Work out the finished part from the listing and answer in its coordinate system (mm). Round coordinates to 2 decimals unless told otherwise and drop trailing zeros. Order: outer loops, then holes, each group sorted by start corner. A loop starts at its lowest first (then second) coordinate and runs counter-clockwise, first axis right, second up. Notation, with made-up numbers: (89.25, -21.5) - (128.25, -21.5) arc R19 cw to (128.25, 8.5) - close; hole circle Ø3 at (61, 45.25). An arc over 180 degrees is marked (long way). Answer in a Markdown table with one row per item.
from build123d import *

# Parameters (mm, degrees)
SKETCH1_R               = 12.5
BOSS_EXTRUDE1_DEPTH     = 900
CHAMFER1_SIZE           = 1
SKETCH2_R               = 3.3
CUT_EXTRUDE1_DEPTH      = 40.5
CUT_EXTRUDE1_DEPTH_BACK = 7


with BuildPart() as part:
    # Sketch1 → Boss-Extrude1 (new body)
    with BuildSketch(Plane.XY):
        with Locations((0, 33)):
            Circle(SKETCH1_R)
        Polygon((-27.5, 0), (-4.75, 0), (-4.75, 6.5), (4.75, 6.5), (4.75, 0), (27.5, 0), (27.5, 6), (10.75, 6), (2.089745962, 21), (-2.089745962, 21), (-10.75, 6), (-27.5, 6), align=None)
    extrude(amount=-BOSS_EXTRUDE1_DEPTH)

    # Chamfer1
    chamfer1_edges = [part.edges().sort_by_distance(p)[0] for p in [
        (4.75, 0, -450),
        (-4.75, 0, -450),
    ]]
    chamfer(chamfer1_edges, length=CHAMFER1_SIZE)

    # Sketch2 → Cut-Extrude1 (cut, two sides)
    with BuildSketch(Plane(origin=(0, 6, 0), x_dir=(1, 0, 0), z_dir=(0, 1, 0))) as cut_extrude1_sk:
        with Locations((17.5, 20)):
            Circle(SKETCH2_R)
        with Locations((-17.5, 20)):
            Circle(SKETCH2_R)
        with Locations((-17.5, 220)):
            Circle(SKETCH2_R)
        with Locations((17.5, 220)):
            Circle(SKETCH2_R)
        with Locations((-17.5, 420)):
            Circle(SKETCH2_R)
        with Locations((17.5, 420)):
            Circle(SKETCH2_R)
        with Locations((-17.5, 620)):
            Circle(SKETCH2_R)
        with Locations((17.5, 620)):
            Circle(SKETCH2_R)
        with Locations((-17.5, 820)):
            Circle(SKETCH2_R)
        with Locations((17.5, 820)):
            Circle(SKETCH2_R)
        with Locations((-17.5, 1020)):
            Circle(SKETCH2_R)
        with Locations((17.5, 1020)):
            Circle(SKETCH2_R)
        with Locations((-17.5, 1220)):
            Circle(SKETCH2_R)
        with Locations((17.5, 1220)):
            Circle(SKETCH2_R)
        with Locations((-17.5, 1420)):
            Circle(SKETCH2_R)
        with Locations((17.5, 1420)):
            Circle(SKETCH2_R)
        with Locations((-17.5, 1620)):
            Circle(SKETCH2_R)
        with Locations((17.5, 1620)):
            Circle(SKETCH2_R)
        with Locations((17.5, 880)):
            Circle(SKETCH2_R)
        with Locations((-17.5, 880)):
            Circle(SKETCH2_R)
    extrude(amount=CUT_EXTRUDE1_DEPTH, mode=Mode.SUBTRACT)
    extrude(cut_extrude1_sk.sketch, amount=-CUT_EXTRUDE1_DEPTH_BACK, mode=Mode.SUBTRACT)


solid = part.part
1) Find the intervals of material crossed by probe 1 along X at (y, z) = (3, -820); probe 2 along X at (y, z) = (3.5, -423); probe 3 along X at (y, z) = (4, -616), in increasing order. Write a range as from..to.
Filled in:
| item | result |
|---|---|
| probe 1 | x = -27.5..-20.8, -14.2..-4.75, 4.75..14.2, 20.8..27.5 |
| probe 2 | x = -27.5..-18.87, -16.13..-4.75, 4.75..16.13, 18.87..27.5 |
| probe 3 | x = -27.5..-4.75, 4.75..27.5 |
2) The mould has two halves that part along Y. Classify faces 1 (the face through (16, 0, -444)), 2 (the face through (-6.445, 13.456, -443.7)), 3 (the face through (0, 18, -900)): released by +Y, released by -Y, zero draft, split by the parting line, or undercut.
Filled in:
| item | result |
|---|---|
| face 1 | released by -Y |
| face 2 | undercut |
| face 3 | zero draft |
3) Each of these flat-tipped pins is pushed along its axis until it touches: pin 1 (7.5 mm diameter, centred on x = 17.5, z = -420, fed in from -Y); pin 2 (1 mm diameter, centred on y = 17.5, z = -129, fed in from -X); pin 3 (6 mm diameter, centred on y = 26.5, z = -428.5, fed in from -X); pin 4 (8.5 mm diameter, centred on x = -19.5, z = -232, fed in from +Y). Where does it stop, or does it pass through?
Filled in:
| item | result |
|---|---|
| pin 1 | stops at y = 0 |
| pin 2 | stops at x = -4.4 |
| pin 3 | stops at x = -12 |
| pin 4 | stops at y = 6 |
4) Find section B-B, the plane y = 32. Give the vertices of the cut face in (x, z), then the cut area to 3 significant figures.
Filled in:
| item | result |
|---|---|
| outline | (-12.46, -900) - (12.46, -900) - (12.46, 0) - (-12.46, 0) - close |
| area | 22,400 mm^2 |
5) Find section A-A, the plane z = -262. Give the vertices of the cut face in (x, y).
Filled in:
| item | result |
|---|---|
| outline | (-27.5, 0) - (-5.75, 0) - (-4.75, 1) - (-4.75, 6.5) - (4.75, 6.5) - (4.75, 1) - (5.75, 0) - (27.5, 0) - (27.5, 6) - (10.75, 6) - (2.26, 20.71) arc R12.5 ccw (long way) to (-2.26, 20.71) - (-10.75, 6) - (-27.5, 6) - close |
